Here's the drawing with two shaded views (mm, measured from the low corner). I have some questions. Give positions to 0.01 mm unless a question says otherwise; leave off trailing zeros. Loops run counter-clockwise (first coordinate to the right, second up) from the corner with the lowest first, then second, coordinate; pieces in that order, holes last. Notation, with made-up numbers: (-9, 45.25) - (8, 45.25) arc R27 cw to (8, 70.25) - close; hole circle Ø9 at (4, 72). An arc over 180 degrees is marked (long way). Answer as a JSON object with one key per item and string values. Group by question number.
Item 1: Suppose I cut it at D-D on y = 4. Write out the boundary of the cut face in (x, z), and give its area (3 significant figures).
Item 2: Suppose I cut it at C-C on x = 0.35. Write out the boundary of the cut face in (y, z), and give its area (3 significant figures).
Item 3: Please list where these lines run through material, in increasing order: L1, parallel to Z at x = 0.45, y = 5; L2, parallel to Y at x = 0.5, z = 15; L3, parallel to Z at x = 0.65, y = 4.25.
Item 4: Suppose I cut it at B-B on z = 15. Write out the boundary of the cut face in (x, y).
Item 5: Thinking about a two-plate mould opening in Y: for the marked faces 1, 2 and 3, which applies, pulls with the +Y half, pulls with the -Y half, needs draft (parallel to the pull), parting line crosses it, or undercut?
Item 6: Suppose I cut it at A-A on y = 5. Write out the boundary of the cut face in (x, z).
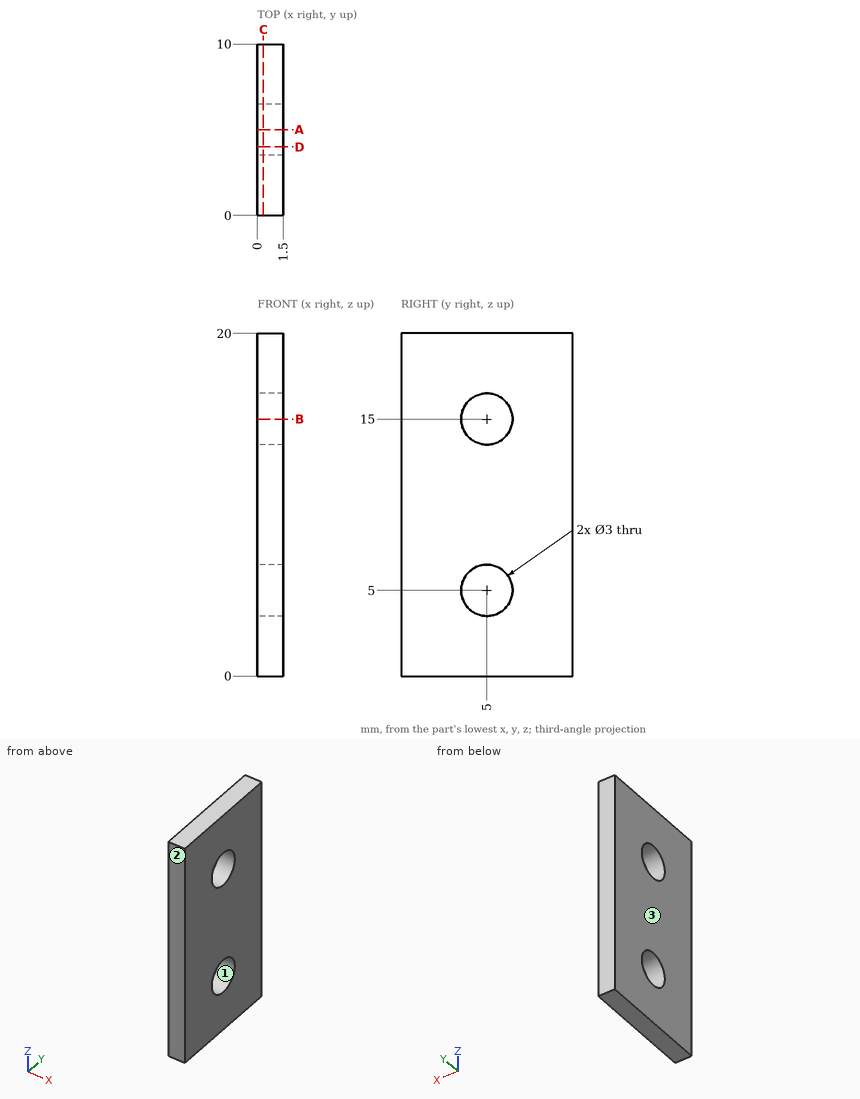
Worked out:
{
 "1": {"outline": "(0, 0) - (1.5, 0) - (1.5, 3.88) - (0, 3.88) - close; (0, 6.12) - (1.5, 6.12) - (1.5, 13.88) - (0, 13.88) - close; (0, 16.12) - (1.5, 16.12) - (1.5, 20) - (0, 20) - close", "area": "23.3 mm2"},
 "2": {"outline": "(0, 0) - (10, 0) - (10, 20) - (0, 20) - close; hole circle Ø3 at (5, 5); hole circle Ø3 at (5, 15)", "area": "186 mm2"},
 "3": {"L1": "z = 0 to 3.5, 6.5 to 13.5, 16.5 to 20", "L2": "y = 0 to 3.5, 6.5 to 10", "L3": "z = 0 to 3.7, 6.3 to 13.7, 16.3 to 20"},
 "4": {"outline": "(0, 0) - (1.5, 0) - (1.5, 3.5) - (0, 3.5) - close; (0, 6.5) - (1.5, 6.5) - (1.5, 10) - (0, 10) - close"},
 "5": {"face 1": "undercut", "face 2": "pulls with the -Y half", "face 3": "needs draft"},
 "6": {"outline": "(0, 0) - (1.5, 0) - (1.5, 3.5) - (0, 3.5) - close; (0, 6.5) - (1.5, 6.5) - (1.5, 13.5) - (0, 13.5) - close; (0, 16.5) - (1.5, 16.5) - (1.5, 20) - (0, 20) - close"}
}
